```python
from build123d import *

# Parameters (mm, degrees)
F1_DEPTH = 28.448
F2_DEPTH = 25.4
F3_DEPTH = 26.924
F4_DEPTH = 26.924
F0_W     = 6.35
F0_H     = 20.115774
F5_DEPTH = 24.638


with BuildPart() as f1:
    # F0 (on Front) → F1 (new body)
    with BuildSketch(Plane.XZ):
        Polygon((0, 0), (0, -19.05), (6.35, -19.05), (82.361273, -19.05), (82.361273, 19.05), (6.35, 19.05), (0, 19.05), align=None)
    extrude(amount=F1_DEPTH)

    # F0 (on Front) → F2 (join)
    with BuildSketch(Plane.XZ):
        Polygon((6.35, 19.05), (82.361273, 19.05), (84.532226, 19.05), (95.708226, 30.226), (69.596, 30.226), (69.596, 39.165774), (6.35, 39.165774), align=None)
        with BuildLine():
            Line((27.993083, 35.814), (63.045083, 35.814))
            ThreePointArc((63.045083, 35.814), (68.633083, 30.226), (63.045083, 24.638))
            Line((63.045083, 24.638), (27.993083, 24.638))
            ThreePointArc((27.993083, 24.638), (22.405083, 30.226), (27.993083, 35.814))
        make_face(mode=Mode.SUBTRACT)
        Polygon((6.35, -19.05), (6.35, -39.165774), (69.596, -39.165774), (69.596, -30.226), (95.708226, -30.226), (84.532226, -19.05), (82.361273, -19.05), align=None)
        with BuildLine():
            ThreePointArc((27.993083, -35.814), (22.405083, -30.226), (27.993083, -24.638))
            Line((27.993083, -24.638), (63.045083, -24.638))
            ThreePointArc((63.045083, -24.638), (68.633083, -30.226), (63.045083, -35.814))
            Line((63.045083, -35.814), (27.993083, -35.814))
        make_face(mode=Mode.SUBTRACT)
    extrude(amount=F2_DEPTH)

    # F0 (on Front) → F3 (join)
    with BuildSketch(Plane.XZ):
        Polygon((69.596, -30.226), (69.596, -39.165774), (104.648, -39.165774), (95.708226, -30.226), align=None)
    extrude(amount=F3_DEPTH)

    # F0 (on Front) → F4 (join)
    with BuildSketch(Plane.XZ):
        Polygon((69.596, 30.226), (95.708226, 30.226), (104.648, 39.165774), (69.596, 39.165774), align=None)
    extrude(amount=F4_DEPTH)

    # F0 (on Front) → F5 (join)
    with BuildSketch(Plane.XZ):
        with Locations((3.175, -29.107887)):
            Rectangle(F0_W, F0_H)
        with Locations((3.175, 29.107887)):
            Rectangle(F0_W, F0_H)
    extrude(amount=F5_DEPTH)


solid = f1.part
```
Work out the finished part from the listing and answer in its coordinate system (mm). A direction names the side the tool comes from. Give positions to 0.01 mm unless a question says otherwise; leave off trailing zeros. Write each loop counter-clockwise with the first axis right and the second up, starting at its lowest first coordinate (ties: lowest second). Pieces come first, ordered by that corner, then holes. Notation, with made-up numbers: (3, 59.25) -> (45, 59.25) arc R15 cw to (45, 76.25) -> close; hole circle Ø11 at (81.5, -23). An arc over 180 degrees is marked (long way). Write item = value, one per line.
Q1. Section A-A on x = 51.5 is taken. Determine the outline of the cut face in (y, z).
Computed values:
outline = (-28.45, -19.05) -> (-25.4, -19.05) -> (-25.4, -24.64) -> (0, -24.64) -> (0, 24.64) -> (-25.4, 24.64) -> (-25.4, 19.05) -> (-28.45, 19.05) -> close; (-25.4, -39.17) -> (0, -39.17) -> (0, -35.81) -> (-25.4, -35.81) -> close; (-25.4, 35.81) -> (0, 35.81) -> (0, 39.17) -> (-25.4, 39.17) -> close
Q2. Flat-ended cylindrical pins translate along their axes: pin 1 Ø16 at (x, z) = (70, 29) entering from -Y; pin 2 Ø0.8 at (y, z) = (-26, -35) entering from -X; pin 3 Ø6 at (y, z) = (-4, -10) entering from +X. Find the tip coordinate at first contact, or state that the pin passes through.
Computed values:
pin_1 = -26.92
pin_2 = 69.6
pin_3 = 82.36
Q3. Section C-C on x = 80 is taken. Determine the outline of the cut face in (y, z), and give its area (3 significant figures).
Computed values:
outline = (-28.45, -19.05) -> (-25.4, -19.05) -> (-25.4, -30.23) -> (-26.92, -30.23) -> (-26.92, -39.17) -> (0, -39.17) -> (0, 39.17) -> (-26.92, 39.17) -> (-26.92, 30.23) -> (-25.4, 30.23) -> (-25.4, 19.05) -> (-28.45, 19.05) -> close
area = 2,130 mm^2
Q4. Section B-B on y = -14.5 is taken. Determine the outline of the cut face in (x, z), and give its area (3 significant figures).
Computed values:
outline = (0, -39.17) -> (104.65, -39.17) -> (84.53, -19.05) -> (82.36, -19.05) -> (82.36, 19.05) -> (84.53, 19.05) -> (104.65, 39.17) -> (0, 39.17) -> close; hole (27.99, -35.81) -> (63.05, -35.81) arc R5.59 ccw to (63.05, -24.64) -> (27.99, -24.64) arc R5.59 ccw to start; hole (27.99, 24.64) -> (63.05, 24.64) arc R5.59 ccw to (63.05, 35.81) -> (27.99, 35.81) arc R5.59 ccw to start
area = 5,960 mm^2
Q5. A tool of negligible diameter and unlimited length cuts with its end or side. For faces 5 (the flat face through (3, -24.638, 29)), 6 (the flat face through (83, -26.924, -35)), 7 (the flat face through (82.361, -14, 0)), 8 (the cylindrical face through (22.406, -12.522, -30.349)), from which of +Z, -Z, +X, -X, +Y, -Y can it reach the whole face along a straight path? Write none if from no direction.
Computed values:
face_5 = +Z, -X, -Y
face_6 = -Z, +X, -X, -Y
face_7 = +X, +Y, -Y
face_8 = +Y, -Y
Q6. Consider line 1 along Z through (x, y) = (50.5, -20); line 2 along Z through (x, y) = (23, -22.5); line 3 along X through (y, z) = (-18.5, 17.5). Determine where each line is inside the solid, lowest interval first.
Computed values:
line_1 = -39.17 to -35.81, -24.64 to 24.64, 35.81 to 39.17
line_2 = -39.17 to -32.73, -27.72 to 27.72, 32.73 to 39.17
line_3 = 0 to 82.36
Q7. Section D-D on z = -27 is taken. Determine the outline of the cut face in (x, y), and give its area (3 significant figures).
Computed values:
outline = (0, -24.64) -> (6.35, -24.64) -> (6.35, -25.4) -> (23.43, -25.4) -> (23.43, 0) -> (0, 0) -> close; (67.61, -25.4) -> (92.48, -25.4) -> (92.48, 0) -> (67.61, 0) -> close
area = 1,220 mm^2
Q8. For a pull along X with two mould halves and no side action, classify faces 1 (the flat face through (45, -13, 35.814)), 2 (the flat face through (41, -27, -19.05)), 3 (the flat face through (0, -14, -1)), 4 (the flat face through (46, -13, 24.638)) as pulls with the +X half, pulls with the -X half, needs draft (parallel to the pull), parting line crosses it, or undercut.
Computed values:
face_1 = undercut
face_2 = needs draft
face_3 = pulls with the -X half
face_4 = undercut
